Read the model definition and answer for the solid it produces. Units are mm, in the model's axes. Face numbers are marked on the shaded views. Round coordinates to 2 decimals unless told otherwise and drop trailing zeros. Write each loop counter-clockwise with the first axis right and the second up, starting at its lowest first coordinate (ties: lowest second). Pieces come first, ordered by that corner, then holes.
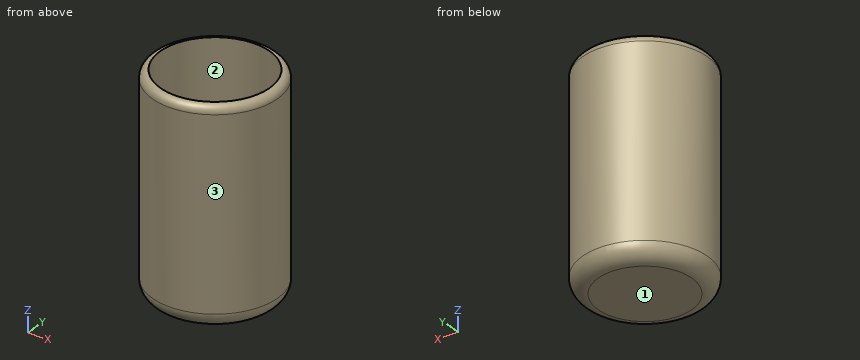
from build123d import *

# Parameters (mm, degrees)
F0_W   = 35
F0_H   = 10
F0_W_2 = 5
F0_H_2 = 125
F2_R   = 4.99999
F3_R   = 10


# Not quite as in the source:
# - a fillet or chamfer is up to 0.001 mm smaller than in the source, because OpenCascade refuses the exact size


with BuildPart() as f1:
    # F0 (on Front) → F1 (revolve)
    with BuildSketch(Plane.XZ):
        with Locations((17.5, 5)):
            Rectangle(F0_W, F0_H)
        with Locations((37.5, 5)):
            Rectangle(F0_W_2, F0_H)
        with Locations((37.5, 72.5)):
            Rectangle(F0_W_2, F0_H_2)
    revolve(axis=Axis((0, 0, 5), (0, 0, -1)))

    # F2 (radius 5 in the source; OpenCascade refuses exactly that, so slightly less here)
    f2_edges = [f1.edges().sort_by_distance(p)[0] for p in [
        (-40, 0, 135),
    ]]
    fillet(f2_edges, radius=F2_R)

    # F3
    f3_edges = [f1.edges().sort_by_distance(p)[0] for p in [
        (-40, 0, 0),
    ]]
    fillet(f3_edges, radius=F3_R)


solid = f1.part
Q1. Flat-ended cylindrical pins translate along their axes: pin 1 Ø12 at (x, z) = (-11, 44.5) entering from -Y; pin 2 Ø2 at (x, z) = (11.5, 118) entering from +Y; pin 3 Ø3 at (x, z) = (31, 21.5) entering from +Y. Find the tip coordinate at first contact, or state that the pin passes through.
Verdict:
pin 1: stops at y = -39.69
pin 2: stops at y = 38.6
pin 3: stops at y = 27.01
Q2. Determine the mould class of the marked faces 1, 2 and 3 for opening direction X: pulls with the +X half, pulls with the -X half, needs draft (parallel to the pull), parting line crosses it, or undercut.
Verdict:
face 1: needs draft
face 2: undercut
face 3: parting line crosses it
Q3. Section C-C (z = 84.5) is taken. Determine the outline of the cut face in (x, y).
Verdict:
outline: circle Ø80 at (0, 0); hole circle Ø70 at (0, 0)
Q4. Straight lines are drawn through the part: probe 1 along Y at (x, z) = (0, 64); probe 2 along Y at (x, z) = (-32, 83). For each, find the intervals that lie inside material, in ascending order.
Verdict:
probe 1: y = -40 to -35, 35 to 40
probe 2: y = -24 to -14.18, 14.18 to 24
